Could you check a few things on this model? Use its own coordinates, in mm. A direction names the side the tool comes from. Give positions to 0.01 mm unless a question says otherwise; leave off trailing zeros. Write each loop counter-clockwise with the first axis right and the second up, starting at its lowest first coordinate (ties: lowest second). Pieces come first, ordered by that corner, then holes. Notation, with made-up numbers: (39.25, 72.5) - (52.25, 72.5) arc R21 ccw to (52.25, 95.5) - close; hole circle Ø8 at (64, -9). An arc over 180 degrees is marked (long way). Answer as CSV lines item,"result". Start each with the question number.
Q1. Imagine slicing it at A-A on x = 0. List the corners of the cut face in (y, z) for me.
Q2. Will these pins go through, and if not, where does the flat tip stop? pin 1 Ø3 at (x, z) = (-2, 11.5) entering from -Y; pin 2 Ø13 at (x, z) = (0, 0) entering from +Y.
Q3. Imagine slicing it at B-B on y = 4.75. List the corners of the cut face in (x, z) for me.
Q4. Imagine slicing it at D-D on z = -16.5. List the corners of the cut face in (x, y) for me, and give its area (3 significant figures).
Q5. If I drill on line 1 along X through (y, z) = (1.25, 0); line 2 along X through (y, z) = (7, -16.5); line 3 along Z through (x, y) = (-13, 5.75), over which ranges is the centre line in solid material (lowest first)?
Q6. Imagine slicing it at C-C on z = -3. List the corners of the cut face in (x, y) for me.
Q7. We'd pull the mould along X, two halves only. Please class faces 3 (the face through (-17.5, 6, 0)), 4 (the face through (0, 7, 23)), 5 (the face through (17.5, 6, 0)): pulls with the +X half, pulls with the -X half, needs draft (parallel to the pull), parting line crosses it, or undercut.
Q8. On a 3-axis mill with a long thin cutter (end or side, diameter ignored), from which of +Z, -Z, +X, -X, +Y, -Y can I reach the whole of each face in a straight line? I mean faces 1 (the face through (15.5, 7, 0)), 2 (the face through (0, 6, -25)). Say none if no direction works.
Autodesk Inventor part; units mm, degrees
ref_plane "РабПлоскость1" through (0, -35, 0) normal (0, 1, 0) x (-1, 0, 0)
ref_plane "РабПлоскость25" through (100, -155, 0) normal (-1, 0, 0) x (0, 0, 1)
ref_plane "РабПлоскость26" through (84, -165, -19) normal (-1, 0, 0) x (0, 0, 1)
sketch "Эскиз130" plane through (0, 0, 0) normal (0, 1, 0) x (-1, 0, 0)
  line L0 (-17.5, 25) -> (17.5, 25)
  line L1 (17.5, 25) -> (17.5, -25)
  line L2 (17.5, -25) -> (-17.5, -25)
  line L3 (-17.5, -25) -> (-17.5, 25)
  line L4 (-17.5, 25) -> (17.5, -25) construction
  line L5 (17.5, 25) -> (-17.5, -25) construction
  point P0 (0, 0)
  dimension "d710" = 50
  dimension "d711" = 35
extrude "Выдавливание115" add sketch "Эскиз130" along normal blind 2
sketch "Эскиз131" plane through (0, 2, 0) normal (0, 1, 0) x (1, 0, 0)
  line L0 (15.5, -23) -> (-15.5, -23)
  line L1 (-15.5, -23) -> (-15.5, 23)
  line L2 (-15.5, 23) -> (15.5, 23)
  line L3 (15.5, 23) -> (15.5, -23)
  line L4 (15.5, -23) -> (-15.5, 23) construction
  line L5 (-15.5, -23) -> (15.5, 23) construction
  line L6 (-17.5, 25) -> (-17.5, -25)
  line L7 (17.5, 25) -> (-17.5, 25)
  line L8 (-17.5, -25) -> (17.5, -25)
  line L9 (17.5, -25) -> (17.5, 25)
  line L10 (-17.5, -25) -> (17.5, -25)
  line L11 (17.5, -25) -> (17.5, 25)
  line L12 (17.5, 25) -> (-17.5, 25)
  line L13 (-17.5, 25) -> (-17.5, -25)
  point P0 (0, 0)
  dimension "d714" = 2
  dimension "d715" = 2
extrude "Выдавливание116" add sketch "Эскиз131" along normal blind 10
sketch "Эскиз132" plane through (0, 2, 0) normal (0, 1, 0) x (1, 0, 0)
  circle A0 centre (0, 0) radius 5
  dimension "d718" = 10
  dimension "d12" = 100
  dimension "d14" = 17
  dimension "d26" = 5
extrude "Выдавливание117" cut sketch "Эскиз132" against normal blind 10
sketch "Эскиз6" plane through (0, -35, -85) normal (0, -1, 0) x (1, 0, 0)
  arc A0 (29.3991, 164.4544) -> (0, 170) centre (-5, 62.7941) ccw
  line L0 (0, 170) -> (0, 0)
  arc A1 (0, 0) -> (29.3991, 5.5456) centre (-5, 107.2059) ccw
  arc A2 (29.3991, 5.5456) -> (100, 85) centre (-5, 107.2059) ccw
  arc A3 (100, 85) -> (29.3991, 164.4544) centre (-5, 62.7941) ccw
  point P0 (0, 85)
sketch "Эскиз114" plane through (2, -165, 82.8837) normal (1, 0, 0) x (0, 0, -1)
  circle A0 centre (120.1897, 5) radius 1
  line L0 (-2.1163, 0) -> (167.8837, 0) construction
  line L1 (82.8837, 0) -> (82.8837, 60.2174) construction
  circle A1 centre (45.5777, 5) radius 1
  point P0 (82.8837, 165)
  dimension "d609" = 2
  dimension "d610" = 37.306
  dimension "d611" = 5
sketch "Эскиз115" plane through (2, -165, 82.8837) normal (1, 0, 0) x (0, 0, -1)
  line L0 (167.7717, 0) -> (0, 0) construction
  line L1 (82.8837, 130) -> (82.8837, 0) construction
  line L2 (63.8837, 0) -> (101.8837, 0)
  line L3 (101.8837, 0) -> (101.8837, 20)
  line L4 (101.8837, 20) -> (63.8837, 20)
  line L5 (63.8837, 20) -> (63.8837, 0)
  line L6 (65.8837, 2) -> (99.8837, 2)
  line L7 (99.8837, 2) -> (99.8837, 18)
  line L8 (99.8837, 18) -> (65.8837, 18)
  line L9 (65.8837, 18) -> (65.8837, 2)
  line L10 (65.8837, 2) -> (99.8837, 18) construction
  line L11 (99.8837, 2) -> (65.8837, 18) construction
  point P0 (82.8837, 165)
  point P1 (145.8837, 0)
  point P2 (82.8837, 20)
  point P3 (82.8837, 10)
  dimension "d614" = 38
  dimension "d615" = 20
  dimension "d616" = 2
  dimension "d617" = 2
  dimension "d618" = 2
sketch "Эскиз116" plane through (0, -165, -85) normal (0, -1, 0) x (1, 0, 0)
  arc A0 (91.9272, 104) -> (2, 167.8837) centre (-5, 62.7941) ccw construction
  arc A1 (97.9549, 85) -> (92.7533, 102) centre (-5, 62.7941) ccw construction
  arc A2 (97.9549, 85) -> (91.9272, 104) centre (-5, 62.7941) ccw construction
  arc A3 (91.9272, 66) -> (97.9549, 85) centre (-5, 107.206) ccw
  line L0 (2, 66) -> (100.2736, 66) construction
  arc A4 (100.2736, 66) -> (97.9549, 85) centre (-5, 62.7941) ccw
  line L1 (91.9272, 66) -> (100.2736, 66)
  point P0 (0, 85)
  point P1 (36.5, 159.5958)
  dimension "d621" = 22.206
sketch "Эскиз117" plane through (2, -165, 82.8837) normal (1, 0, 0) x (0, 0, -1)
  line L0 (101.8837, 20) -> (101.8837, 0)
  line L1 (63.8837, 20) -> (101.8837, 20)
  line L2 (63.8837, 0) -> (63.8837, 20)
  line L3 (63.8837, 0) -> (101.8837, 0)
  point P0 (82.8837, 165)
sketch "Эскиз118" plane through (0, -165, -85) normal (0, -1, 0) x (1, 0, 0)
  line L0 (2, 66) -> (2, 104)
  line L1 (2, 66) -> (91.9272, 66)
  arc A0 (91.9272, 66) -> (97.9549, 85) centre (-5, 107.206) ccw
  line L2 (97.9549, 85) -> (100, 85)
  arc A1 (100, 85) -> (94.0968, 104) centre (-5, 62.7941) ccw
  line L3 (2, 104) -> (94.0968, 104)
  line L4 (2, 104) -> (4, 104)
  line L5 (4, 104) -> (4, 66)
  line L6 (4, 66) -> (2, 66)
  line L7 (2, 66) -> (2, 104)
  point P0 (0, 85)
  dimension "d626" = 2
sketch "Эскиз119" plane through (0, -165, -85) normal (0, -1, 0) x (1, 0, 0)
  arc A0 (100, 85) -> (94.0968, 104) centre (-5, 62.7941) ccw construction
  line L0 (4, 104) -> (4, 66) construction
  line L1 (4, 85) -> (65.3021, 85) construction
  arc A1 (94.0968, 66) -> (100, 85) centre (-5, 107.2059) ccw
  arc A2 (91.9272, 66) -> (97.9549, 85) centre (-5, 107.206) ccw construction
  line L2 (100, 85) -> (97.9549, 85)
  line L3 (94.0968, 66) -> (91.9272, 66)
  arc A3 (91.9272, 66) -> (97.9549, 85) centre (-5, 107.206) ccw
  point P0 (0, 85)
sketch "Эскиз120" plane through (4, -147, 17) normal (0, -1, 0) x (1, 0, 0)
  line L0 (0, 0) -> (2, 0)
  line L1 (2, 0) -> (2, -34)
  line L2 (2, -34) -> (0, -34)
  line L3 (0, -34) -> (0, 0)
  point P0 (-4, -17)
  dimension "d631" = 2
sketch "Эскиз121" plane through (0, 0, 0) normal (1, 0, 0) x (0, 1, 0)
  line L0 (-145, -19) -> (-145, 19) construction
  line L1 (-165, -19) -> (-145, -19) construction
  line L2 (-165, 19) -> (-165, -19) construction
  line L3 (-145, 19) -> (-165, 19) construction
  line L4 (-158, -19) -> (-152, -19)
  line L5 (-152, -19) -> (-152, -25)
  line L6 (-152, -25) -> (-158, -25)
  line L7 (-158, -25) -> (-158, -19)
  circle A0 centre (-155, -22) radius 1
  line L8 (-158, 25) -> (-152, 25)
  line L9 (-152, 25) -> (-152, 19)
  line L10 (-152, 19) -> (-158, 19)
  line L11 (-158, 19) -> (-158, 25)
  circle A1 centre (-155, 22) radius 1
  line L12 (-155, 19) -> (-155, -19) construction
  point P0 (0, 0)
  dimension "d634" = 6
  dimension "d635" = 6
  dimension "d636" = 2
  dimension "d637" = 3
  dimension "d638" = 3
  dimension "d639" = 6
  dimension "d640" = 6
  dimension "d641" = 2
  dimension "d642" = 3
  dimension "d643" = 3
sketch "Эскиз122" plane through (0, -158, 19) normal (0, -1, 0) x (1, 0, 0)
  line L0 (0, 0) -> (0, 6)
  line L1 (0, 0) -> (4, 0)
  line L2 (6, 0) -> (4, 0)
  line L3 (6, 6) -> (6, 0)
  line L4 (0, 6) -> (6, 6)
  line L5 (0, -44) -> (0, -38)
  line L6 (0, -44) -> (6, -44)
  line L7 (6, -38) -> (6, -44)
  line L8 (4, -38) -> (6, -38)
  line L9 (0, -38) -> (4, -38)
  line L10 (0, 6) -> (4, 6)
  line L11 (4, 6) -> (4, -44)
  line L12 (4, -44) -> (0, -44)
  line L13 (0, -44) -> (0, 6)
  line L14 (0, -44) -> (6, -44)
  point P0 (0, -19)
  dimension "d646" = 4
sketch "Эскиз123" plane through (0, -165, -85) normal (0, -1, 0) x (1, 0, 0)
  line L0 (32, 66) -> (34, 66)
  line L1 (34, 66) -> (34, 63)
  line L2 (34, 63) -> (32, 63)
  line L3 (32, 63) -> (32, 66)
  line L4 (4, 104) -> (4, 66)
  line L5 (94.0968, 66) -> (4, 66)
  line L6 (32, 107) -> (34, 107)
  line L7 (34, 107) -> (34, 104)
  line L8 (34, 104) -> (32, 104)
  line L9 (32, 104) -> (32, 107)
  line L10 (4, 104) -> (94.0968, 104)
  line L11 (36.5, 107) -> (38.5, 107)
  line L12 (38.5, 107) -> (38.5, 104)
  line L13 (38.5, 104) -> (36.5, 104)
  line L14 (36.5, 104) -> (36.5, 107)
  line L15 (36.5, 66) -> (38.5, 66)
  line L16 (38.5, 66) -> (38.5, 63)
  line L17 (38.5, 63) -> (36.5, 63)
  line L18 (36.5, 63) -> (36.5, 66)
  point P0 (0, 85)
  dimension "d650" = 30
  dimension "d651" = 2
  dimension "d652" = 3
  dimension "d653" = 2
  dimension "d654" = 3
  dimension "d655" = 2
  dimension "d656" = 3
  dimension "d657" = 2
  dimension "d658" = 3
  dimension "d659" = 30
  dimension "d660" = 2.5
  dimension "d661" = 2.5
sketch "Эскиз124" plane through (36.5, -145, -19) normal (0, 0, 1) x (1, 0, 0)
  line L0 (0, 0) -> (2, 0)
  line L1 (2, 0) -> (2, 2)
  line L2 (0, 2) -> (2, 2)
  line L3 (0, 0) -> (0, 2)
  line L4 (-4.5, 0) -> (-2.5, 0)
  line L5 (-2.5, 0) -> (-2.5, 2)
  line L6 (-4.5, 2) -> (-2.5, 2)
  line L7 (-4.5, 0) -> (-4.5, 2)
  point P0 (-36.5, 145)
  dimension "d667" = 2
  dimension "d668" = 9.5
  dimension "d669" = 10
sketch "Эскиз126" plane through (0, -165, -85) normal (0, -1, 0) x (1, 0, 0)
  circle A0 centre (16, 79) radius 1
  circle A1 centre (16, 91) radius 1
  line L0 (4, 104) -> (4, 66)
  line L1 (4, 85) -> (100.0263, 85) construction
  circle A2 centre (31, 79) radius 1
  circle A3 centre (31, 91) radius 1
  circle A4 centre (71, 75) radius 1
  circle A5 centre (71, 95) radius 1
  point P0 (0, 85)
  dimension "d674" = 2
  dimension "d675" = 2
  dimension "d676" = 12
  dimension "d677" = 12
  dimension "d678" = 6
  dimension "d679" = 2
  dimension "d680" = 2
  dimension "d681" = 12
  dimension "d683" = 27
  dimension "d684" = 6
  dimension "d685" = 2
  dimension "d686" = 2
  dimension "d689" = 67
  dimension "d690" = 10
  dimension "d697" = 20
sketch "Эскиз127" plane through (0, -165, -85) normal (0, -1, 0) x (1, 0, 0)
  circle A0 centre (71, 75) radius 1 construction
  circle A1 centre (31, 79) radius 1 construction
  circle A2 centre (16, 79) radius 1 construction
  circle A3 centre (16, 91) radius 1 construction
  circle A4 centre (31, 91) radius 1 construction
  circle A5 centre (71, 95) radius 1 construction
  arc A6 (32, 64) -> (34, 64) centre (33, 64) ccw construction
  line L0 (34, 64) -> (34, 66) construction
  line L1 (36.5, 66) -> (34, 66) construction
  line L2 (36.5, 66) -> (36.5, 64) construction
  arc A7 (36.5, 64) -> (38.5, 64) centre (37.5, 64) ccw construction
  line L3 (38.5, 64) -> (38.5, 66) construction
  line L4 (94.0968, 66) -> (38.5, 66) construction
  arc A8 (94.0968, 66) -> (100, 85) centre (-5, 107.2059) ccw
  arc A9 (100, 85) -> (94.0968, 104) centre (-5, 62.7941) ccw
  line L5 (38.5, 104) -> (94.0968, 104) construction
  line L6 (38.5, 104) -> (38.5, 106) construction
  arc A10 (38.5, 106) -> (36.5, 106) centre (37.5, 106) ccw construction
  line L7 (36.5, 106) -> (36.5, 104) construction
  line L8 (34, 104) -> (36.5, 104) construction
  line L9 (34, 104) -> (34, 106) construction
  arc A11 (34, 106) -> (32, 106) centre (33, 106) ccw construction
  line L10 (32, 106) -> (32, 104) construction
  line L11 (4, 104) -> (32, 104) construction
  line L12 (4, 104) -> (4, 66) construction
  line L13 (32, 66) -> (4, 66) construction
  line L14 (32, 66) -> (32, 64) construction
  line L15 (4, 85) -> (100, 85) construction
  line L16 (4, 84) -> (99.7835, 84)
  line L17 (4, 86) -> (99.7835, 86)
  line L18 (4, 86) -> (4, 84)
  point P0 (0, 85)
  dimension "d693" = 2
  dimension "d694" = 1
sketch "Эскиз128" plane through (84, -165, -19) normal (-1, 0, 0) x (0, 0, 1)
  line L0 (-7, 0) -> (46, 0)
  line L1 (46, 0) -> (46, 24)
  line L2 (46, 24) -> (-7, 24)
  line L3 (-7, 24) -> (-7, 0)
  point P0 (19, 165)
  point P1 (0, 0)
  dimension "d699" = 53
  dimension "d700" = 24
  dimension "d701" = 7
sketch "Эскиз129" plane through (38.5, -145, 19) normal (0, 1, 0) x (1, 0, 0)
  arc A0 (45.5, 48) -> (45.5, -10) centre (79.9093, 19) ccw
  line L0 (45.5, 48) -> (45.5, -10)
  line L1 (45.5, 0) -> (45.5, 38)
  line L2 (0, 0) -> (45.5, 0)
  point P0 (-38.5, 19)
  dimension "d707" = 10
  dimension "d708" = 10
  dimension "d709" = 45
  dimension "d10" = 170
  dimension "d15" = 4
  dimension "d16" = 35
  dimension "d97" = 2
properties part number "тело"
Conclusion:
1,outline,"(0, -25) - (12, -25) - (12, -23) - (2, -23) - (2, -5) - (0, -5) - close; (0, 5) - (2, 5) - (2, 23) - (12, 23) - (12, 25) - (0, 25) - close"
2,pin 1,"y = 0"
2,pin 2,"y = 2"
3,outline,"(-17.5, -25) - (17.5, -25) - (17.5, 25) - (-17.5, 25) - close; hole (-15.5, -23) - (15.5, -23) - (15.5, 23) - (-15.5, 23) - close"
4,outline,"(-17.5, 0) - (17.5, 0) - (17.5, 12) - (15.5, 12) - (15.5, 2) - (-15.5, 2) - (-15.5, 12) - (-17.5, 12) - close"
4,area,"110 mm^2"
5,line 1,"-17.5 to -5, 5 to 17.5"
5,line 2,"-17.5 to -15.5, 15.5 to 17.5"
5,line 3,"-25 to -23, 23 to 25"
6,outline,"(-17.5, 0) - (-4, 0) - (-4, 2) - (-15.5, 2) - (-15.5, 12) - (-17.5, 12) - close; (4, 0) - (17.5, 0) - (17.5, 12) - (15.5, 12) - (15.5, 2) - (4, 2) - close"
7,face 3,"pulls with the -X half"
7,face 4,"undercut"
7,face 5,"pulls with the +X half"
8,face 1,"+Y"
8,face 2,"-Z, +X, -X, +Y, -Y"
